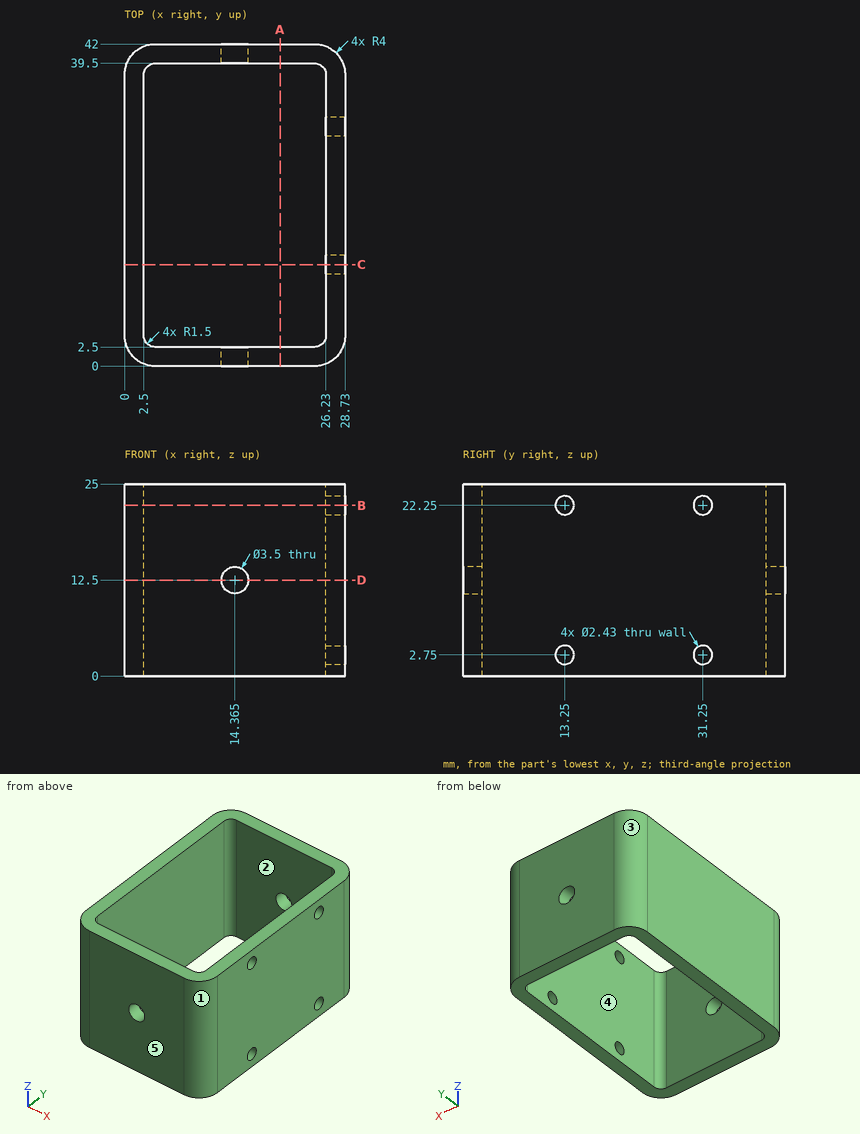
Design review of the part shown in the three views and the two pictorial views. Dimensions are in mm from the part's minimum x, y and z. A direction names the side the tool comes from. Coordinates: 2 decimals unless noted, no trailing zeros. Write each loop counter-clockwise with the first axis right and the second up, starting at its lowest first coordinate (ties: lowest second). Pieces come first, ordered by that corner, then holes.
(1) Add section A-A on x = 20.25. Give the boundary of the cut face in (y, z), then the cut area to 3 significant figures.
(2) For pin 1 Ø4.5 at (x, z) = (14.365, 12.5) entering from -Y; pin 2 Ø5 at (x, y) = (21.5, 27) entering from +Z; pin 3 Ø1.5 at (y, z) = (13.25, 22.25) entering from +X, all flat-tipped, find the tip position at first contact; note any pin that passes through.
(3) Wall thickness on probe 1 along Z at (x, y) = (28.25, 31.25) (3 decimals); probe 2 along X at (y, z) = (34, 22.5); probe 3 along Y at (x, z) = (11.5, 3.5): over which ranges is each line inside the solid? List them lowest first.
(4) Add section C-C on y = 13.25. Give the boundary of the cut face in (x, z) (3 decimals).
(5) Tool access review of the marked faces 4 and 5: name each direction out of +Z, -Z, +X, -X, +Y, -Y from which nothing blocks a thin tool from reaching the whole face with its end or side.
(6) Add section D-D on z = 12.5. Give the boundary of the cut face in (x, y) (3 decimals).
(7) The part is to be moulded in two halves that separate along X. For the marked faces 1, 2 and 3, say which applies: +X half, -X half, draft (parallel to the pull), parting line (faces both ways), or undercut.
(8) Add section B-B on z = 22.25. Give the boundary of the cut face in (x, y) (3 decimals).
Answer sheet:
1. outline: (0, 0) - (2.5, 0) - (2.5, 25) - (0, 25) - close; (39.5, 0) - (42, 0) - (42, 25) - (39.5, 25) - close
1. area: 125 mm2
2. pin 1: stops at y = 0
2. pin 2: passes through
2. pin 3: stops at x = 2.5
3. probe 1: z = 0 to 1.535, 3.965 to 21.035, 23.465 to 25
3. probe 2: x = 0 to 2.5, 26.23 to 28.73
3. probe 3: y = 0 to 2.5, 39.5 to 42
4. outline: (0, 0) - (2.5, 0) - (2.5, 25) - (0, 25) - close; (26.23, 0) - (28.73, 0) - (28.73, 1.535) - (26.23, 1.535) - close; (26.23, 3.965) - (28.73, 3.965) - (28.73, 21.035) - (26.23, 21.035) - close; (26.23, 23.465) - (28.73, 23.465) - (28.73, 25) - (26.23, 25) - close
5. face 4: +Z, -Z
5. face 5: +Z, -Z, +X, -X, -Y
6. outline: (0, 4) arc R4 ccw to (4, 0) - (12.615, 0) - (12.615, 2.5) - (4, 2.5) arc R1.5 cw to (2.5, 4) - (2.5, 38) arc R1.5 cw to (4, 39.5) - (12.615, 39.5) - (12.615, 42) - (4, 42) arc R4 ccw to (0, 38) - close; (16.115, 0) - (24.73, 0) arc R4 ccw to (28.73, 4) - (28.73, 38) arc R4 ccw to (24.73, 42) - (16.115, 42) - (16.115, 39.5) - (24.73, 39.5) arc R1.5 cw to (26.23, 38) - (26.23, 4) arc R1.5 cw to (24.73, 2.5) - (16.115, 2.5) - close
7. face 1: +X half
7. face 2: undercut
7. face 3: -X half
8. outline: (0, 4) arc R4 ccw to (4, 0) - (24.73, 0) arc R4 ccw to (28.73, 4) - (28.73, 12.035) - (26.23, 12.035) - (26.23, 4) arc R1.5 cw to (24.73, 2.5) - (4, 2.5) arc R1.5 cw to (2.5, 4) - (2.5, 38) arc R1.5 cw to (4, 39.5) - (24.73, 39.5) arc R1.5 cw to (26.23, 38) - (26.23, 32.465) - (28.73, 32.465) - (28.73, 38) arc R4 ccw to (24.73, 42) - (4, 42) arc R4 ccw to (0, 38) - close; (26.23, 14.465) - (28.73, 14.465) - (28.73, 30.035) - (26.23, 30.035) - close
